from build123d import *

# Parameters (mm, degrees)
F0_R     = 50
F0_R_2   = 5
F0_R_3   = 26
F0_R_4   = 22
F0_R_5   = 20
F1_DEPTH = 6
F2_R     = 26
F2_R_2   = 22
F3_DEPTH = 3
F5_R     = 26
F5_R_2   = 22
F6_DEPTH = 3
F7_SIZE  = 0.6


with BuildPart() as f1:
    # F0 (on Front) → F1 (new body, symmetric)
    with BuildSketch(Plane.XZ):
        Circle(F0_R)
        with Locations((-32.9089653438, -19)):
            Circle(F0_R_2, mode=Mode.SUBTRACT)
        with Locations((0, -38)):
            Circle(F0_R_2, mode=Mode.SUBTRACT)
        with Locations((32.9089653438, -19)):
            Circle(F0_R_2, mode=Mode.SUBTRACT)
        with Locations((-32.9089653438, 19)):
            Circle(F0_R_2, mode=Mode.SUBTRACT)
        Circle(F0_R_3, mode=Mode.SUBTRACT)
        with Locations((32.9089653438, 19)):
            Circle(F0_R_2, mode=Mode.SUBTRACT)
        with Locations((0, 38)):
            Circle(F0_R_2, mode=Mode.SUBTRACT)
        Circle(F0_R_3)
        Circle(F0_R_4, mode=Mode.SUBTRACT)
        Circle(F0_R_4)
        Circle(F0_R_5, mode=Mode.SUBTRACT)
    extrude(amount=F1_DEPTH, both=True)

    # F2 (on face) → F3 (cut)
    with BuildSketch(Plane.XZ.offset(6)):
        Circle(F2_R)
        Circle(F2_R_2, mode=Mode.SUBTRACT)
    extrude(amount=-F3_DEPTH, mode=Mode.SUBTRACT)

    # F5 (on face) → F6 (cut)
    with BuildSketch(Plane(origin=(0, 6, 0), x_dir=(-1, 0, 0), z_dir=(0, 1, 0))):
        Circle(F5_R)
        Circle(F5_R_2, mode=Mode.SUBTRACT)
    extrude(amount=-F6_DEPTH, mode=Mode.SUBTRACT)

    # F7
    f7_edges = [f1.edges().sort_by_distance(p)[0] for p in [
        (-50, 6, 0),
        (50, 0, 0),
        (-50, -6, 0),
    ]]
    chamfer(f7_edges, length=F7_SIZE)


solid = f1.part
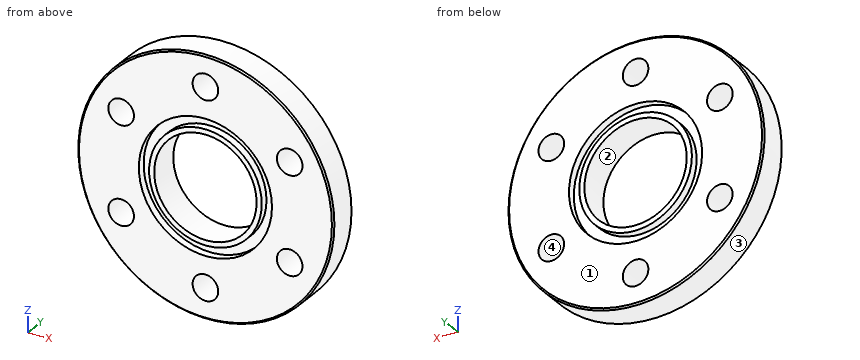
The listing builds one solid part. Answer for the finished solid, in the listing's coordinates (mm). Face numbers are marked on the shaded views. Round coordinates to 2 decimals unless told otherwise and drop trailing zeros. Order: outer loops, then holes, each group sorted by start corner. A loop starts at its lowest first (then second) coordinate and runs counter-clockwise, first axis right, second up. Notation, with made-up numbers: (-6, 0) -> (3, 0) arc R25 cw to (3, 25) -> close; hole circle Ø7 at (-38.5, 32). An arc over 180 degrees is marked (long way). Put each result on its own line as item: value.
Q1. Consider line 1 along Z through (x, y) = (0, 1.25); line 2 along Z through (x, y) = (0, 5.35); line 3 along X through (y, z) = (-5, 16). Determine where each line is inside the solid, lowest interval first.
Results list:
line 1: -50 to -43, -33 to -20, 20 to 33, 43 to 50
line 2: -50 to -43, -33 to -26, -22 to -20, 20 to 22, 26 to 33, 43 to 50
line 3: -47.37 to -36.91, -28.91 to -20.49, -15.1 to -12, 12 to 15.1, 20.49 to 28.91, 36.91 to 47.37
Q2. Section A-A, the plane z = 0 is taken. Write down the section's boundary in (x, y), and give its area (3 significant figures).
Results list:
outline: (-50, -5.4) -> (-49.4, -6) -> (-26, -6) -> (-26, -3) -> (-22, -3) -> (-22, -6) -> (-20, -6) -> (-20, 6) -> (-22, 6) -> (-22, 3) -> (-26, 3) -> (-26, 6) -> (-49.4, 6) -> (-50, 5.4) -> close; (20, -6) -> (22, -6) -> (22, -3) -> (26, -3) -> (26, -6) -> (49.4, -6) -> (50, -5.4) -> (50, 5.4) -> (49.4, 6) -> (26, 6) -> (26, 3) -> (22, 3) -> (22, 6) -> (20, 6) -> close
area: 671 mm^2
Q3. Section B-B, the plane y = -1.75 is taken. Write down the section's boundary in (x, z), and give its area (3 significant figures).
Results list:
outline: circle Ø100 at (0, 0); hole circle Ø10 at (-32.91, -19); hole circle Ø10 at (-32.91, 19); hole circle Ø40 at (0, 0); hole circle Ø10 at (0, -38); hole circle Ø10 at (0, 38); hole circle Ø10 at (32.91, -19); hole circle Ø10 at (32.91, 19)
area: 6,130 mm^2
Q4. Each of these flat-tipped pins is pushed along its axis until it touches: P1, Ø16, axis at x = 32.91, z = -19, coming from the -Y side; P2, Ø4, axis at y = -1.5, z = 9.5, coming from the -X side; P3, Ø3, axis at x = 2.5, y = 1, coming from the -Z side; P4, Ø6, axis at x = -7.5, y = 0, coming from the +Z side. Where does it stop, or does it pass through?
Results list:
P1: y = -6
P2: x = -49.43
P3: z = -49.99
P4: z = 49.8
Q5. Determine the mould class of the marked faces 1, 2, 3 and 4 for opening direction X: pulls with the +X half, pulls with the -X half, needs draft (parallel to the pull), parting line crosses it, or undercut.
Results list:
face 1: needs draft
face 2: undercut
face 3: parting line crosses it
face 4: undercut
Q6. Section C-C, the plane x = 0 is taken. Count the separate pieces of the cut face and the enclosed holes in it, and give its area (3 significant figures).
Results list:
separate pieces: 4
enclosed holes: 0
area: 431 mm^2
